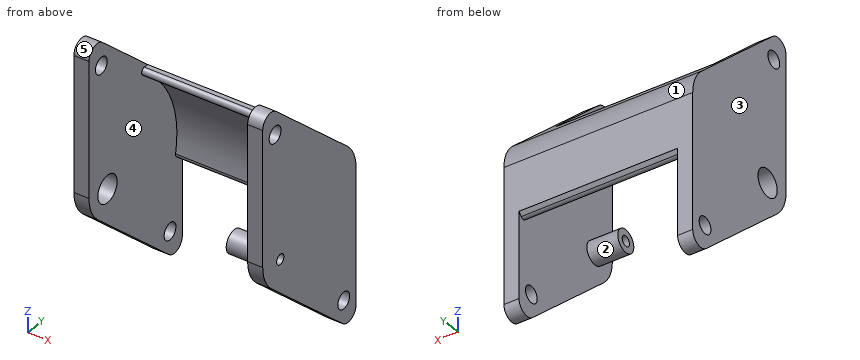
from build123d import *

# Parameters (mm, degrees)
SKETCH4_R            = 3.6
THICKBASE_DEPTH      = 4
MIDDLE_DEPTH         = 42
THINBASE_DEPTH       = 4
SKETCH8_R            = 1.35
RETAINERSCREW_DEPTH  = 4
SKETCH9_R            = 3
SKETCH9_R_2          = 1.35
SPACER_DEPTH         = 8.2
SKETCH15_W           = 42
SKETCH15_H           = 16
CUT_EXTRUDE_H1_DEPTH = 77.519145025
SKETCH17_W           = 42
SKETCH17_H           = 16
CUT_EXTRUDE_H2_DEPTH = 75.830901411
FILLET_R1_R          = 1
FILLET_R2_R          = 1
SKETCH18_R           = 2.21
SIDESCREWS_DEPTH     = 71.502298398


with BuildPart() as part:
    # Sketch4 → ThickBase (new body)
    with BuildSketch(Plane(origin=(0, 0, 0), x_dir=(0, 0, -1), z_dir=(1, 0, 0))):
        with BuildLine():
            Line((-14.01318338, 16.550216151), (21.822267157, 16.550216151))
            ThreePointArc((21.822267157, 16.550216151), (24.561793845, 14.77291543), (24.055345362, 11.546878503))
            Line((24.055345362, 11.546878503), (0.125176293, -15.12757601))
            ThreePointArc((0.125176293, -15.12757601), (-3.242753458, -17.581539475), (-7.318417722, -18.449783849))
            Line((-7.318417722, -18.449783849), (-43.153868259, -18.449783849))
            ThreePointArc((-43.153868259, -18.449783849), (-45.893394947, -16.672483128), (-45.386946464, -13.446446201))
            Line((-45.386946464, -13.446446201), (-21.456777395, 13.228008312))
            ThreePointArc((-21.456777395, 13.228008312), (-18.088847644, 15.681971777), (-14.01318338, 16.550216151))
        make_face()
        with Locations((-5.952745457, -11.509649573)):
            Circle(SKETCH4_R, mode=Mode.SUBTRACT)
    extrude(amount=THICKBASE_DEPTH)

    # Sketch5 → Middle (add)
    with BuildSketch(Plane(origin=(4, 0, 0), x_dir=(0, 0, -1), z_dir=(1, 0, 0))):
        with BuildLine():
            Line((15.945305194, 2.506787856), (24.055345362, 11.546878503))
            ThreePointArc((24.055345362, 11.546878503), (24.561793845, 14.77291543), (21.822267157, 16.550216151))
            Line((21.822267157, 16.550216151), (-14.01318338, 16.550216151))
            ThreePointArc((-14.01318338, 16.550216151), (-18.088847644, 15.681971777), (-21.456777395, 13.228008312))
            Line((-21.456777395, 13.228008312), (-45.386946464, -13.446446201))
            ThreePointArc((-45.386946464, -13.446446201), (-45.893394947, -16.672483128), (-43.153868259, -18.449783849))
            Line((-43.153868259, -18.449783849), (-31.009075531, -18.449783849))
            ThreePointArc((-31.009075531, -18.449783849), (-16.549356077, 12.232654103), (15.945305194, 2.506787856))
        make_face()
    extrude(amount=MIDDLE_DEPTH)

    # Sketch7 → ThinBase (add)
    with BuildSketch(Plane(origin=(46, 0, 0), x_dir=(0, 0, -1), z_dir=(1, 0, 0))):
        with BuildLine():
            ThreePointArc((15.945305194, 2.506787856), (-16.549356077, 12.232654103), (-31.009075531, -18.449783849))
            Line((-31.009075531, -18.449783849), (-7.318417722, -18.449783849))
            ThreePointArc((-7.318417722, -18.449783849), (-3.242753458, -17.581539475), (0.125176293, -15.12757601))
            Line((0.125176293, -15.12757601), (15.945305194, 2.506787856))
        make_face()
        with BuildLine():
            Line((-43.153868259, -18.449783849), (-31.009075531, -18.449783849))
            ThreePointArc((-31.009075531, -18.449783849), (-16.549356077, 12.232654103), (15.945305194, 2.506787856))
            Line((15.945305194, 2.506787856), (24.055345362, 11.546878503))
            ThreePointArc((24.055345362, 11.546878503), (24.561793845, 14.77291543), (21.822267157, 16.550216151))
            Line((21.822267157, 16.550216151), (-14.01318338, 16.550216151))
            ThreePointArc((-14.01318338, 16.550216151), (-18.088847644, 15.681971777), (-21.456777395, 13.228008312))
            Line((-21.456777395, 13.228008312), (-45.386946464, -13.446446201))
            ThreePointArc((-45.386946464, -13.446446201), (-45.893394947, -16.672483128), (-43.153868259, -18.449783849))
        make_face()
    extrude(amount=THINBASE_DEPTH)

    # Sketch8 → RetainerScrew (cut)
    with BuildSketch(Plane(origin=(50, 0, 0), x_dir=(0, 0, -1), z_dir=(1, 0, 0))):
        with Locations((-5.789718886, -11.874919798)):
            Circle(SKETCH8_R)
    extrude(amount=-RETAINERSCREW_DEPTH, mode=Mode.SUBTRACT)

    # Sketch9 → Spacer (add)
    with BuildSketch(Plane.ZY.offset(-46)):
        with Locations(Location((5.789718886, -11.874919798, 0), (0, 0, 180))):
            Circle(SKETCH9_R)
        with Locations(Location((5.789718886, -11.874919798, 0), (0, 0, 180))):
            Circle(SKETCH9_R_2, mode=Mode.SUBTRACT)
    extrude(amount=SPACER_DEPTH)

    # Sketch15 → Cut-Extrude H1 (cut, through all)
    with BuildSketch(Plane(origin=(0, 16.550216151, 0), x_dir=(1, 0, 0), z_dir=(0, 1, 0))):
        with Locations((25, -38.153868259)):
            Rectangle(SKETCH15_W, SKETCH15_H)
    extrude(amount=-CUT_EXTRUDE_H1_DEPTH, mode=Mode.SUBTRACT)

    # Sketch17 → Cut-Extrude H2 (cut, through all)
    with BuildSketch(Plane(origin=(0, 16.564225392, 18.463792524), x_dir=(1, 0, 0), z_dir=(0, 0.6677792161146302, 0.7443594014488768))):
        with Locations((25, 19.65868724)):
            Rectangle(SKETCH17_W, SKETCH17_H)
    extrude(amount=-CUT_EXTRUDE_H2_DEPTH, mode=Mode.SUBTRACT)

    # Fillet R1
    fillet_r1_edges = [part.edges().sort_by_distance(p)[0] for p in [
        (25, -2.007502678, 30.153868259),
    ]]
    fillet(fillet_r1_edges, radius=FILLET_R1_R)

    # Fillet R2
    fillet_r2_edges = [part.edges().sort_by_distance(p)[0] for p in [
        (25, 12.850019915, -3.135248981),
    ]]
    fillet(fillet_r2_edges, radius=FILLET_R2_R)

    # Sketch18 → SideScrews (cut, through all)
    with BuildSketch(Plane(origin=(50, 0, 0), x_dir=(0, 0, -1), z_dir=(1, 0, 0))):
        with Locations((-39.501166009, -13.819518143)):
            Circle(SKETCH18_R)
        with Locations((18.169564907, 11.919950445)):
            Circle(SKETCH18_R)
    extrude(amount=-SIDESCREWS_DEPTH, mode=Mode.SUBTRACT)


solid = part.part
Model file for the job. Use its own axes, mm. Face numbers are marked on the shaded views. A direction names the side the tool comes from. Give positions to 0.01 mm unless a question says otherwise; leave off trailing zeros. Loops run counter-clockwise (first coordinate to the right, second up) from the corner with the lowest first, then second, coordinate; pieces in that order, holes last. Notation, with made-up numbers: (47.5, 25) -> (102.5, 25) arc R5 ccw to (102.5, 30) -> close; hole circle Ø5 at (55, 8). An arc over 180 degrees is marked (long way). Use a Markdown table: item, result. Add a question column.
(1) Slice it at A-A on x = 41.5. List the corners of the cut face in (y, z), and give its area (3 significant figures).
(2) Mould opens along X. For the marked faces 3, 4 and 5 say: +X half, -X half, draft (parallel to the pull), parting line (faces both ways), or undercut.
(3) Drop flat-ended pins along their axis: pin 1 Ø4.5 at (y, z) = (-11.87, 5.79) entering from +X; pin 2 Ø8 at (x, y) = (20.5, 6.5) entering from -Z; pin 3 Ø1 at (x, y) = (43, 9.5) entering from +Z; pin 4 Ø1.4 at (x, y) = (33, 2.5) entering from +Z. Give the stop position or say it passes through.
(4) Tool access for the marked faces 1 and 2: list every direction of +Z, -Z, +X, -X, +Y, -Y with a clear straight run to the whole face (end or side of a thin tool).
(5) Slice it at B-B on z = -6.5. List the corners of the cut face in (x, y).
(6) Wall check: line 1 along Y through (x, z) = (38, 6); line 2 along X through (y, z) = (3, 13.5); line 3 along Z through (x, y) = (39.5, -13). Give the ranges that are in metal, low to high.
(7) Slice it at C-C on y = -3.5. List the corners of the cut face in (x, z), and give its area (3 significant figures).
(8) Slice it at D-D on y = 4.5. List the corners of the cut face in (x, z).
Filled sheet:
| question | item | result |
|---|---|---|
| 1 | outline | circle Ø6 at (-11.87, 5.79); (1.79, 28.29) arc R26 cw to (14, 0.93) arc R1 ccw to (15.73, 0.07) -> (16.55, 0.99) -> (16.55, 14.01) arc R10 ccw to (13.23, 21.46) -> (3.53, 30.15) -> (2.3, 30.15) arc R1 ccw to start; hole circle Ø2.7 at (-11.87, 5.79) |
| 1 | area | 114 mm2 |
| 2 | face 3 | -X half |
| 2 | face 4 | undercut |
| 2 | face 5 | draft |
| 3 | pin 1 | x = 50 |
| 3 | pin 2 | z = 19.79 |
| 3 | pin 3 | z = 25.25 |
| 3 | pin 4 | z = 30.15 |
| 4 | face 1 | +Z, +X, -X, +Y |
| 4 | face 2 | -X |
| 5 | outline | (0, -8.02) -> (4, -8.02) -> (4, 16.55) -> (0, 16.55) -> close; (46, -8.02) -> (50, -8.02) -> (50, 16.55) -> (46, 16.55) -> close |
| 6 | line 1 | -14.87 to -13.21, -10.54 to -8.88, 14.49 to 16.55 |
| 6 | line 2 | 0 to 4, 46 to 50 |
| 6 | line 3 | 3.01 to 5.04, 6.54 to 8.57 |
| 7 | outline | (0, -10.56) -> (4, -10.56) -> (4, 36.46) -> (0, 36.46) -> close; (46, -10.56) -> (50, -10.56) -> (50, 36.46) -> (46, 36.46) -> close |
| 7 | area | 376 mm2 |
| 8 | outline | (0, -17.73) -> (4, -17.73) -> (4, 26.44) -> (46, 26.44) -> (46, -17.73) -> (50, -17.73) -> (50, 29.29) -> (0, 29.29) -> close |
